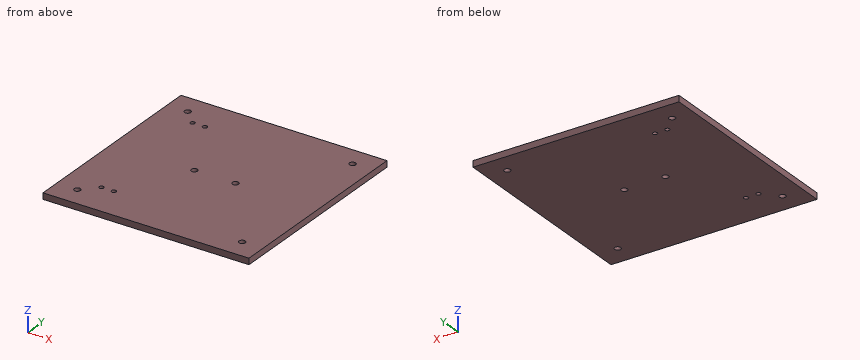
from build123d import *

# Parameters (mm, degrees)
F0_W     = 100
F0_H     = 100
F1_DEPTH = 3
F2_R     = 1.5
F3_DEPTH = 3.001
F4_R     = 1.1
F5_DEPTH = 3.001
F6_R     = 1.5
F7_DEPTH = 3.001


with BuildPart() as f1:
    # F0 (on Top) → F1 (new body)
    with BuildSketch(Plane.XY):
        with Locations((50, 50)):
            Rectangle(F0_W, F0_H)
    extrude(amount=F1_DEPTH)

    # F2 (on face) → F3 (cut, through all)
    with BuildSketch(Plane.XY.offset(3)):
        with Locations((10, 90)):
            Circle(F2_R)
        with Locations((90, 90)):
            Circle(F2_R)
        with Locations((90, 10)):
            Circle(F2_R)
        with Locations((10, 10)):
            Circle(F2_R)
    extrude(amount=-F3_DEPTH, mode=Mode.SUBTRACT)

    # F4 (on face) → F5 (cut, through all)
    with BuildSketch(Plane.XY.offset(3)):
        with Locations((17, 83)):
            Circle(F4_R)
        with Locations((23, 83)):
            Circle(F4_R)
        with Locations((17, 17)):
            Circle(F4_R)
        with Locations((23, 17)):
            Circle(F4_R)
    extrude(amount=-F5_DEPTH, mode=Mode.SUBTRACT)

    # F6 (on face) → F7 (cut, through all)
    with BuildSketch(Plane.XY.offset(3)):
        with Locations((40, 50)):
            Circle(F6_R)
        with Locations((60, 50)):
            Circle(F6_R)
    extrude(amount=-F7_DEPTH, mode=Mode.SUBTRACT)


solid = f1.part
Can you work these out from the model? Positions are in its coordinate system, mm. Coordinates: 2 decimals unless noted, no trailing zeros. Write each loop counter-clockwise with the first axis right and the second up, starting at its lowest first coordinate (ties: lowest second). Pieces come first, ordered by that corner, then holes.
Q1. Imagine slicing it at C-C, the plane y = 50. List the corners of the cut face in (x, z) for me, plus the area to 3 significant figures.
Results found:
outline: (0, 0) - (38.5, 0) - (38.5, 3) - (0, 3) - close; (41.5, 0) - (58.5, 0) - (58.5, 3) - (41.5, 3) - close; (61.5, 0) - (100, 0) - (100, 3) - (61.5, 3) - close
area: 282 mm2
Q2. Please list where these lines run through material, in increasing order: L1, parallel to Y at x = 23, z = 2.2; L2, parallel to X at y = 83, z = 1.7; L3, parallel to Y at x = 10, z = 1.15.
Results found:
L1: y = 0 to 15.9, 18.1 to 81.9, 84.1 to 100
L2: x = 0 to 15.9, 18.1 to 21.9, 24.1 to 100
L3: y = 0 to 8.5, 11.5 to 88.5, 91.5 to 100
Q3. Imagine slicing it at B-B, the plane x = 60. List the corners of the cut face in (y, z) for me.
Results found:
outline: (0, 0) - (48.5, 0) - (48.5, 3) - (0, 3) - close; (51.5, 0) - (100, 0) - (100, 3) - (51.5, 3) - close
Q4. For P1, Ø1.3, axis at x = 17, y = 17, coming from the -Z side, with a flat end and sliding along its axis, tell me the tip position at first contact or that it passes through.
Results found:
P1: passes through
Q5. Imagine slicing it at A-A, the plane x = 90. List the corners of the cut face in (y, z) for me.
Results found:
outline: (0, 0) - (8.5, 0) - (8.5, 3) - (0, 3) - close; (11.5, 0) - (88.5, 0) - (88.5, 3) - (11.5, 3) - close; (91.5, 0) - (100, 0) - (100, 3) - (91.5, 3) - close
